The model under review builds one solid part; all positions refer to its coordinate system, in mm. Face numbers are marked on the shaded views. A direction names the side the tool comes from. Round coordinates to 2 decimals unless told otherwise and drop trailing zeros. Loops run counter-clockwise (first coordinate to the right, second up) from the corner with the lowest first, then second, coordinate; pieces in that order, holes last. Notation, with made-up numbers: M 40,73 L 96,73 A26 cw 96,110 Z; hole C -12,59.25 d10. An arc over 180 degrees is marked long. Answer as a JSON object with one key per item and string values. Group by question number.
Item 1: Consider section B-B (y = 3). Give the boundary of the cut face in (x, z).
Item 2: Consider section D-D (x = -7). Give the boundary of the cut face in (y, z).
Item 3: Consider section A-A (z = 2.25). Give the boundary of the cut face in (x, y).
Item 4: To check wall thickness, follow line 1 (Z direction, x = -1.25, y = 2.5); line 2 (X direction, y = 4, z = 4.25); line 3 (Y direction, x = -2.75, z = 10.5). State the ranges of each line that lie inside material, in increasing order.
Item 5: Consider section C-C (x = -5.5). Give the boundary of the cut face in (y, z).
Item 6: Insertion check: P1, Ø4, axis at x = -2, z = 2, coming from the -Y side; P2, Ø6, axis at y = 7.5, z = 6.5, coming from the -X side; P3, Ø1, axis at y = 4, z = 6, coming from the -X side. Each pin has a flat end and moves straight along its axis. Give the tip position at first contact, or say it passes through.
Item 7: Tool access review of the marked faces 4 and 5: name each direction out of +Z, -Z, +X, -X, +Y, -Y from which nothing blocks a thin tool from reaching the whole face with its end or side.
Item 8: The part is to be moulded in two halves that separate along Y. For the marked faces 1, 2 and 3, say which applies: +Y half, -Y half, draft (parallel to the pull), parting line (faces both ways), or undercut.
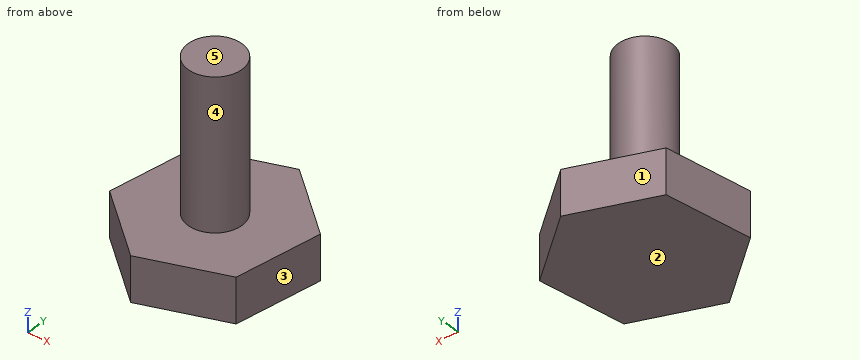
```python
from build123d import *

# Parameters (mm, degrees)
BOSS_EXTRU_1_DEPTH = 3
ESQUISSE2_R        = 1.8
BOSS_EXTRU_2_DEPTH = 10


with BuildPart() as part:
    # Esquisse1 → Boss.-Extru.1 (new body)
    with BuildSketch(Plane.XY):
        Polygon((0.090746241, 0.209409856), (1.049578601, 5.902736989), (-3.401571147, 9.579773737), (-8.811553256, 7.563483353), (-9.770385617, 1.870156221), (-5.319235869, -1.806880528), align=None)
    extrude(amount=BOSS_EXTRU_1_DEPTH)

    # Esquisse2 → Boss.-Extru.2 (add)
    with BuildSketch(Plane.XY.offset(3)):
        with Locations((-4.360403508, 3.886446605)):
            Circle(ESQUISSE2_R)
    extrude(amount=BOSS_EXTRU_2_DEPTH)


solid = part.part
```
Geometry results:
{
 "1": {"outline": "M -9.58,0 L 0.56,0 L 0.56,3 L -2.79,3 L -2.79,13 L -5.93,13 L -5.93,3 L -9.58,3 Z"},
 "2": {"outline": "M -0.42,0 L 8.24,0 L 8.24,3 L -0.42,3 Z"},
 "3": {"outline": "M -9.77,1.87 L -5.32,-1.81 L 0.09,0.21 L 1.05,5.9 L -3.4,9.58 L -8.81,7.56 Z"},
 "4": {"line 1": "z = 0 to 3", "line 2": "x = -6.16 to -2.56", "line 3": "y = 3.08 to 4.69"},
 "5": {"outline": "M -1.66,0 L 8.8,0 L 8.8,3 L 5.28,3 L 5.28,13 L 2.49,13 L 2.49,3 L -1.66,3 Z"},
 "6": {"P1": "stops at y = -1.32", "P2": "stops at x = -6.05", "P3": "stops at x = -6.16"},
 "7": {"face 4": "+Z", "face 5": "+Z, +X, -X, +Y, -Y"},
 "8": {"face 1": "+Y half", "face 2": "draft", "face 3": "-Y half"}
}
